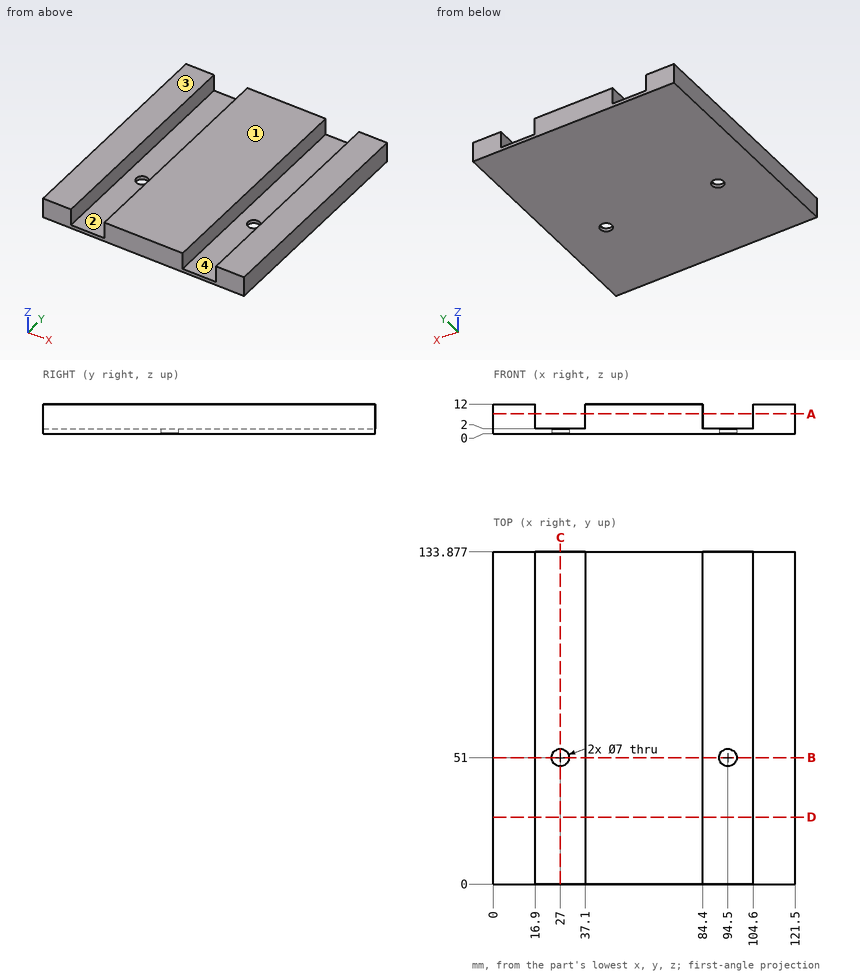
Source: three-view drawing plus pictorial views. Frame: mm from the lowest corner of the part. A direction names the side the tool comes from. Round coordinates to 2 decimals unless told otherwise and drop trailing zeros. Loops run counter-clockwise (first coordinate to the right, second up) from the corner with the lowest first, then second, coordinate; pieces in that order, holes last.
1. Contact query for flat-ended pins moving along their axis: pin 1 (16 mm diameter, centred on x = 97, y = 97.5, fed in from +Z); pin 2 (16 mm diameter, centred on x = 25.5, y = 73.5, fed in from +Z); pin 3 (6.5 mm diameter, centred on x = 94.5, y = 51, fed in from +Z). Output: stop coordinate, or through.
2. Ray query, L1, parallel to X at y = 12, z = 10.25; L2, parallel to Y at x = 27, z = 0.65; L3, parallel to Z at x = 99.5, y = 50.5. Return the intervals inside material, ascending.
3. Mould query, pull axis X, two halves, no side actions, for the marked faces 1 and 2. Classes: released by +X, released by -X, zero draft, split by the parting line, or undercut.
4. Section query D-D on y = 27. Output: boundary loops of the cut face in (x, z), and give its area (3 significant figures).
5. Section query C-C on x = 27. Output: boundary loops of the cut face in (y, z), and give its area (3 significant figures).
6. Section query B-B on y = 51. Output: boundary loops of the cut face in (x, z), and give its area (3 significant figures).
7. Access query for the marked faces 3 and 4. Directions: +Z, -Z, +X, -X, +Y, -Y. A direction counts if a zero-diameter tool reaches every point of the face in a straight line with its end or side. Return the directions, or none.
8. Section query A-A on z = 8. Output: boundary loops of the cut face in (x, y), and give its area (3 significant figures).
Answers below:
1. pin 1: stops at z = 12
1. pin 2: stops at z = 2
1. pin 3: passes through
2. L1: x = 0 to 16.9, 37.1 to 84.4, 104.6 to 121.5
2. L2: y = 0 to 47.5, 54.5 to 133.88
2. L3: z = 0 to 2
3. face 1: zero draft
3. face 2: undercut
4. outline: (0, 0) - (121.5, 0) - (121.5, 12) - (104.6, 12) - (104.6, 2) - (84.4, 2) - (84.4, 12) - (37.1, 12) - (37.1, 2) - (16.9, 2) - (16.9, 12) - (0, 12) - close
4. area: 1,050 mm2
5. outline: (0, 0) - (47.5, 0) - (47.5, 2) - (0, 2) - close; (54.5, 0) - (133.88, 0) - (133.88, 2) - (54.5, 2) - close
5. area: 254 mm2
6. outline: (0, 0) - (23.5, 0) - (23.5, 2) - (16.9, 2) - (16.9, 12) - (0, 12) - close; (30.5, 0) - (91, 0) - (91, 2) - (84.4, 2) - (84.4, 12) - (37.1, 12) - (37.1, 2) - (30.5, 2) - close; (98, 0) - (121.5, 0) - (121.5, 12) - (104.6, 12) - (104.6, 2) - (98, 2) - close
6. area: 1,030 mm2
7. face 3: +Z, +X, -X, +Y, -Y
7. face 4: +Z, +Y, -Y
8. outline: (0, 0) - (16.9, 0) - (16.9, 133.88) - (0, 133.88) - close; (37.1, 0) - (84.4, 0) - (84.4, 133.88) - (37.1, 133.88) - close; (104.6, 0) - (121.5, 0) - (121.5, 133.88) - (104.6, 133.88) - close
8. area: 10,900 mm2
